Input: part model. Units: mm. Frame: model coordinates. Face numbers are marked on the shaded views. A direction names the side the tool comes from. Coordinates: 2 decimals unless noted, no trailing zeros. Order: outer loops, then holes, each group sorted by start corner. A loop starts at its lowest first (then second) coordinate and runs counter-clockwise, first axis right, second up. Notation, with made-up numbers: (51.5, -2) -> (103.5, -2) arc R20 ccw to (103.5, 17) -> close; hole circle Ø8 at (39, 53). An arc over 180 degrees is marked (long way). Use CSV: the item, a comma, the result in double quotes. Start each with the question number.
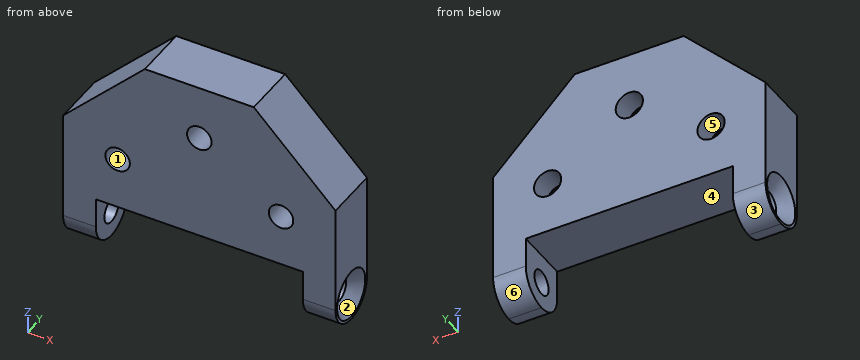
```python
from build123d import *

# Parameters (mm, degrees)
BOSS_EXTRUDE1_DEPTH                     = 10
FILLET1_R                               = 5
CBORE_FOR_M5_HEX_HEAD_BOLT1_D           = 4.5
CBORE_FOR_M5_HEX_HEAD_BOLT1_DEPTH       = 10
CBORE_FOR_M5_HEX_HEAD_BOLT1_CBORE_D     = 5
CBORE_FOR_M5_HEX_HEAD_BOLT1_CBORE_DEPTH = 4.2
CBORE_FOR_M5_HEX_HEAD_BOLT1_TIP         = 1.351936393
CHAMFER1_SIZE                           = 15


with BuildPart() as part:
    # Sketch1 → Boss-Extrude1 (new body)
    with BuildSketch(Plane(origin=(0, 0, 0), x_dir=(1, 0, 0), z_dir=(0, 1, 0))):
        Polygon((-25, 20), (-25, -20), (25, -20), (25, 20), (19, 20), (19, 9.5), (-19, 9.5), (-19, 20), align=None)
    extrude(amount=BOSS_EXTRUDE1_DEPTH)

    # Fillet1
    fillet1_edges = [part.edges().sort_by_distance(p)[0] for p in [
        (22, 10, -20),
        (22, 0, -20),
        (-22, 0, -20),
        (-22, 10, -20),
    ]]
    fillet(fillet1_edges, radius=FILLET1_R - 0.0001)  # a hair under: the kernel refuses the full size

    # Sketch3 → CSK for M4 SFHCS1 (revolve, cut)
    with BuildSketch(Plane(origin=(25, 5, -15), x_dir=(0, 0, -1), z_dir=(0, 1, 0))):
        Polygon((0, 0), (0, 11.351936393), (2.25, 10), (2.25, 2.23), (4.48, 0), align=None)
    csk_for_m4_sfhcs1 = revolve(axis=Axis((31.35, 5, -15), (-1, 0, 0)), mode=Mode.SUBTRACT)

    # Mirror1: CSK for M4 SFHCS1 across plane
    add(csk_for_m4_sfhcs1.mirror(Plane(origin=(0, 0, 0), x_dir=(0, 0, 1), z_dir=(1, 0, 0))), mode=Mode.SUBTRACT)

    # CBORE for M5 Hex Head Bolt1
    with Locations(Plane(origin=(0, 10, 0), x_dir=(1, 0, 0), z_dir=(0, 1, 0))):
        with Locations((-15, 0), (15, 0), (0, -10)):
            CounterBoreHole(CBORE_FOR_M5_HEX_HEAD_BOLT1_D / 2, CBORE_FOR_M5_HEX_HEAD_BOLT1_CBORE_D / 2, CBORE_FOR_M5_HEX_HEAD_BOLT1_CBORE_DEPTH, depth=CBORE_FOR_M5_HEX_HEAD_BOLT1_DEPTH)
            with Locations((0, 0, -(CBORE_FOR_M5_HEX_HEAD_BOLT1_DEPTH + CBORE_FOR_M5_HEX_HEAD_BOLT1_TIP / 2))):  # 118° drill point
                Cone(0, CBORE_FOR_M5_HEX_HEAD_BOLT1_D / 2, CBORE_FOR_M5_HEX_HEAD_BOLT1_TIP, mode=Mode.SUBTRACT)

    # Chamfer1
    chamfer1_edges = [part.edges().sort_by_distance(p)[0] for p in [
        (25, 5, 20),
        (-25, 5, 20),
    ]]
    chamfer(chamfer1_edges, length=CHAMFER1_SIZE)


solid = part.part
```
1. Section B-B on x = 0. Return loops of the section in (y, z), then the cut area to 3 significant figures.
2. Access query for the marked faces 4, 5 and 6. Directions: +Z, -Z, +X, -X, +Y, -Y. A direction counts if a zero-diameter tool reaches every point of the face in a straight line with its end or side. Return the directions, or none.
3. Material intervals for line 1 along Y through (x, z) = (21.45, -15); line 2 along X through (y, z) = (8.4, 10); line 3 along X through (y, z) = (3.45, 10), sorted ascending.
4. Section C-C on z = 10. Return loops of the section in (x, y), then the cut area to 3 significant figures.
5. Section D-D on y = 2. State how many separate pieces and enclosed holes the cut face has, then the cut area to 3 significant figures.
6. Section A-A on z = 0. Return loops of the section in (x, y).
7. Contact query for flat-ended pins moving along their axis: P1, Ø5.5, axis at x = -16, z = 1, coming from the +Y side; P2, Ø6, axis at y = 5, z = -15, coming from the -X side; P3, Ø3, axis at x = 19, y = 2, coming from the +Z side; P4, Ø3, axis at y = 4, z = -17, coming from the +X side. Output: stop coordinate, or through.
8. Pull-direction query (Y, two-part tool) for the marked faces 1, 2 and 3; classes: released by +Y, released by -Y, zero draft, split by the parting line, or undercut.
Values follow:
1,outline,"(0, -9.5) -> (10, -9.5) -> (10, 7.5) -> (5.8, 7.5) -> (5.8, 7.75) -> (0, 7.75) -> close; (0, 12.25) -> (5.8, 12.25) -> (5.8, 12.5) -> (10, 12.5) -> (10, 20) -> (0, 20) -> close"
1,area,"248 mm2"
2,face 4,"-Z, +Y, -Y"
2,face 5,"+Y"
2,face 6,"-Z, +X, -X, +Y"
3,line 1,"y = 0 to 2.75, 7.25 to 10"
3,line 2,"x = -20 to -2.5, 2.5 to 20"
3,line 3,"x = -20 to -2.25, 2.25 to 20"
4,outline,"(-20, 0) -> (-2.25, 0) -> (-2.25, 5.8) -> (-2.5, 5.8) -> (-2.5, 10) -> (-20, 10) -> close; (2.25, 0) -> (20, 0) -> (20, 10) -> (2.5, 10) -> (2.5, 5.8) -> (2.25, 5.8) -> close"
4,area,"353 mm2"
5,separate pieces,"1"
5,enclosed holes,"3"
5,area,"1,300 mm2"
6,outline,"(-25, 0) -> (-17.25, 0) -> (-17.25, 5.8) -> (-17.5, 5.8) -> (-17.5, 10) -> (-25, 10) -> close; (-12.75, 0) -> (12.75, 0) -> (12.75, 5.8) -> (12.5, 5.8) -> (12.5, 10) -> (-12.5, 10) -> (-12.5, 5.8) -> (-12.75, 5.8) -> close; (17.25, 0) -> (25, 0) -> (25, 10) -> (17.5, 10) -> (17.5, 5.8) -> (17.25, 5.8) -> close"
7,P1,"stops at y = 10"
7,P2,"stops at x = -23.52"
7,P3,"stops at z = 12.5"
7,P4,"stops at x = 24.26"
8,face 1,"zero draft"
8,face 2,"undercut"
8,face 3,"released by +Y"
